For this review, use the dimensioned drawing (mm, ordinates from the lowest corner) and the shaded views. A direction names the side the tool comes from. Coordinates: 2 decimals unless noted, no trailing zeros. Write each loop counter-clockwise with the first axis right and the second up, starting at its lowest first coordinate (ties: lowest second). Pieces come first, ordered by that corner, then holes. Notation, with made-up numbers: (67, 87.5) - (118, 87.5) arc R33 cw to (118, 124.5) - close; hole circle Ø6 at (74, 71). An arc over 180 degrees is marked (long way). One line per item, written item: value.
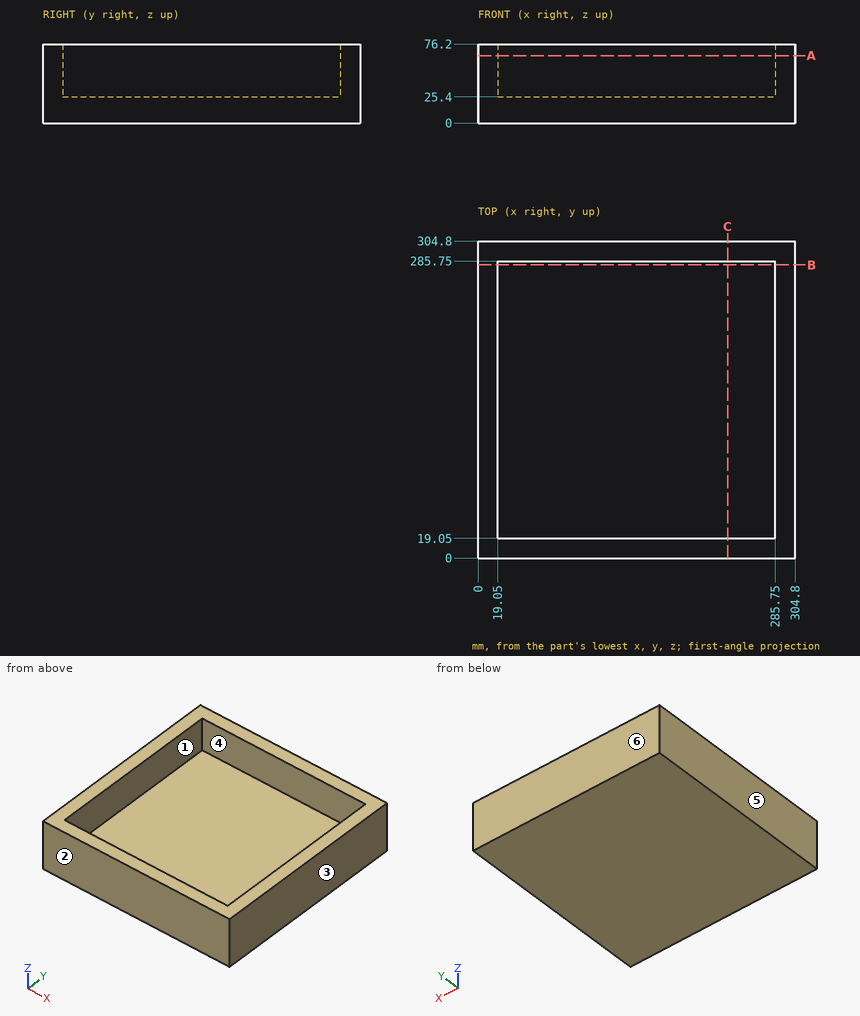
1. Insertion check: pin 1 Ø1 at (x, y) = (195, 254.5) entering from +Z. The pin has a flat end and moves straight along its axis. Give the tip position at first contact, or say it passes through.
Answer block:
pin 1: stops at z = 25.4
2. Consider section A-A, the plane z = 65. Write out the cut boundary in (x, y).
Answer block:
outline: (0, 0) - (304.8, 0) - (304.8, 304.8) - (0, 304.8) - close; hole (19.05, 19.05) - (285.75, 19.05) - (285.75, 285.75) - (19.05, 285.75) - close
3. Mouldability with a two-part tool opening along X and no side actions: class the marked faces 3, 4, 5 and 6 as released by +X, released by -X, zero draft, split by the parting line, or undercut.
Answer block:
face 3: released by +X
face 4: undercut
face 5: released by -X
face 6: zero draft
4. Wall thickness on line 1 along Y through (x, z) = (87, 54.5); line 2 along Z through (x, y) = (263, 63): over which ranges is each line inside the solid? List them lowest first.
Answer block:
line 1: y = 0 to 19.05, 285.75 to 304.8
line 2: z = 0 to 25.4
5. For the marked faces 1 and 2, list the 3-axis set-ups (+Z, -Z, +X, -X, +Y, -Y) from which the entire face can be reached by the end or side of a thin tool; tool diameter is ignored.
Answer block:
face 1: +Z
face 2: +Z, -Z, +X, -X, -Y
6. Consider section B-B, the plane y = 282. Write out the cut boundary in (x, z).
Answer block:
outline: (0, 0) - (304.8, 0) - (304.8, 76.2) - (285.75, 76.2) - (285.75, 25.4) - (19.05, 25.4) - (19.05, 76.2) - (0, 76.2) - close
